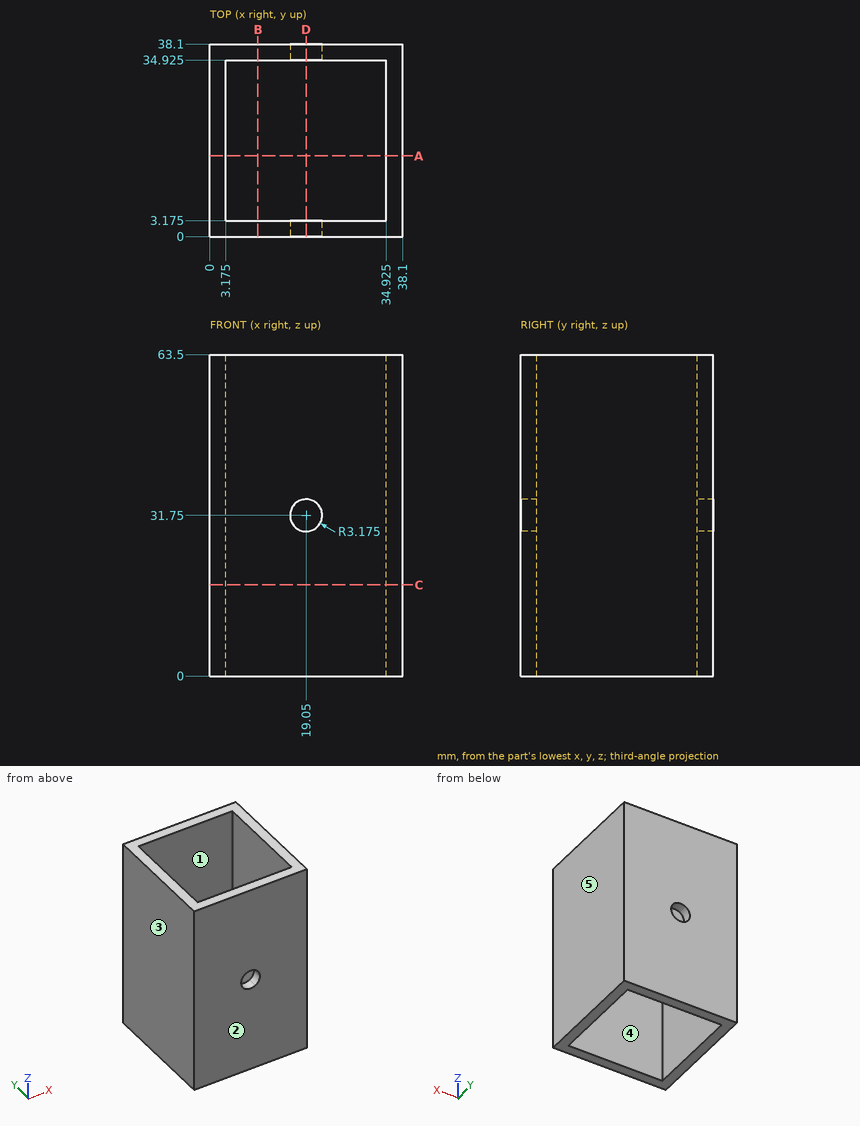
Input: dimensioned drawing with shaded views. Units: mm. Origin: part minimum x, y, z. A direction names the side the tool comes from. Coordinates: 2 decimals unless noted, no trailing zeros. Order: outer loops, then holes, each group sorted by start corner. A loop starts at its lowest first (then second) coordinate and runs counter-clockwise, first axis right, second up. Notation, with made-up numbers: (-24.75, 33) - (-15.75, 33) arc R17 cw to (-15.75, 56) - close; hole circle Ø8 at (-26, 58). An arc over 180 degrees is marked (long way). One line per item, written item: value.
1) Cut plane D-D on x = 19.05. Output: boundary loops of the cut face in (y, z) (3 decimals).
Computed values:
outline: (0, 0) - (3.175, 0) - (3.175, 28.575) - (0, 28.575) - close; (0, 34.925) - (3.175, 34.925) - (3.175, 63.5) - (0, 63.5) - close; (34.925, 0) - (38.1, 0) - (38.1, 28.575) - (34.925, 28.575) - close; (34.925, 34.925) - (38.1, 34.925) - (38.1, 63.5) - (34.925, 63.5) - close
2) Ray query, line 1 (X direction, y = 27, z = 38.5) (3 decimals). Return the intervals inside material, ascending. Write a range as [from, to].
Computed values:
line 1: x = [0, 3.175], [34.925, 38.1]
3) Reachability of the marked faces 4 and 5 from +Z, -Z, +X, -X, +Y, -Y: full face, straight path, thin tool, end or side. Return the list, or none.
Computed values:
face 4: +Z, -Z
face 5: +Z, -Z, +X, +Y, -Y
4) Cut plane A-A on y = 16. Output: boundary loops of the cut face in (x, z) (3 decimals), plus the area to 3 significant figures.
Computed values:
outline: (0, 0) - (3.175, 0) - (3.175, 63.5) - (0, 63.5) - close; (34.925, 0) - (38.1, 0) - (38.1, 63.5) - (34.925, 63.5) - close
area: 403 mm^2
5) Cut plane C-C on z = 18. Output: boundary loops of the cut face in (x, y) (3 decimals), plus the area to 3 significant figures.
Computed values:
outline: (0, 0) - (38.1, 0) - (38.1, 38.1) - (0, 38.1) - close; hole (3.175, 3.175) - (34.925, 3.175) - (34.925, 34.925) - (3.175, 34.925) - close
area: 444 mm^2
6) Mould query, pull axis X, two halves, no side actions, for the marked faces 1, 2 and 3. Classes: released by +X, released by -X, zero draft, split by the parting line, or undercut.
Computed values:
face 1: undercut
face 2: zero draft
face 3: released by -X
